CAD build for the part. Positions are in the model's coordinates, mm. Give positions to 0.01 mm unless a question says otherwise; leave off trailing zeros. Order: outer loops, then holes, each group sorted by start corner. A loop starts at its lowest first (then second) coordinate and runs counter-clockwise, first axis right, second up.
from build123d import *

# Parameters (mm, degrees)
BOSS_EXTRU_1_DEPTH = 2


with BuildPart() as part:
    # Esquisse1 → Boss.-Extru.1 (new body)
    with BuildSketch(Plane.XY):
        with BuildLine():
            Line((-875.748326024, -75.185778964), (-878.248326024, -75.185778964))
            Line((-878.248326024, -75.185778964), (-878.248326024, -67.185778964))
            Line((-878.248326024, -67.185778964), (-875.748326024, -67.185778964))
            Line((-875.748326024, -67.185778964), (-851.698326024, -67.185778964))
            ThreePointArc((-851.698326024, -67.185778964), (-849.970412013, -66.63818863), (-848.873290676, -65.195321078))
            Line((-848.873290676, -65.195321078), (-847.673290676, -61.837321078))
            ThreePointArc((-847.673290676, -61.837321078), (-847.542390805, -61.340074755), (-847.498326024, -60.827778964))
            Line((-847.498326024, -60.827778964), (-847.498326024, -56.827778964))
            ThreePointArc((-847.498326024, -56.827778964), (-847.538821892, -56.336520083), (-847.659216217, -55.858523838))
            Line((-847.659216217, -55.858523838), (-848.859216217, -52.343523838))
            ThreePointArc((-848.859216217, -52.343523838), (-849.95301307, -50.872721036), (-851.698326024, -50.312778964))
            Line((-851.698326024, -50.312778964), (-875.748326024, -50.312778964))
            Line((-875.748326024, -50.312778964), (-878.248326024, -50.312778964))
            Line((-878.248326024, -50.312778964), (-878.248326024, -40.935651694))
            Line((-878.248326024, -40.935651694), (-875.748326024, -40.935651694))
            Line((-875.748326024, -40.935651694), (-871.748326024, -40.935651694))
            Line((-871.748326024, -40.935651694), (-871.748326024, -31.558524425))
            Line((-871.748326024, -31.558524425), (-875.748326024, -31.558524425))
            Line((-875.748326024, -31.558524425), (-878.248326024, -31.558524425))
            Line((-878.248326024, -31.558524425), (-878.248326024, -22.181397155))
            Line((-878.248326024, -22.181397155), (-875.748326024, -22.181397155))
            Line((-875.748326024, -22.181397155), (-617.248326024, -22.181397155))
            Line((-617.248326024, -22.181397155), (-614.748326024, -22.181397155))
            Line((-614.748326024, -22.181397155), (-614.748326024, -31.558524425))
            Line((-614.748326024, -31.558524425), (-617.248326024, -31.558524425))
            Line((-617.248326024, -31.558524425), (-621.248326024, -31.558524425))
            Line((-621.248326024, -31.558524425), (-621.248326024, -40.935651694))
            Line((-621.248326024, -40.935651694), (-617.248326024, -40.935651694))
            Line((-617.248326024, -40.935651694), (-614.748326024, -40.935651694))
            Line((-614.748326024, -40.935651694), (-614.748326024, -50.312778964))
            Line((-614.748326024, -50.312778964), (-621.248326024, -50.312778964))
            Line((-621.248326024, -50.312778964), (-621.248326024, -67.185778964))
            Line((-621.248326024, -67.185778964), (-617.248326024, -67.185778964))
            Line((-617.248326024, -67.185778964), (-614.748326024, -67.185778964))
            Line((-614.748326024, -67.185778964), (-614.748326024, -75.185778964))
            Line((-614.748326024, -75.185778964), (-617.248326024, -75.185778964))
            Line((-617.248326024, -75.185778964), (-875.748326024, -75.185778964))
        make_face()
    extrude(amount=-BOSS_EXTRU_1_DEPTH)


solid = part.part
1. Wall check: line 1 (X direction, y = -35, z = -0.65); line 2 (X direction, y = -62, z = -1.2). Give the ranges that are in metal, low to high.
2. Saw through at B-B on z = -0.6. Give the cut face in (x, y), plus the area to 3 significant figures.
3. Pin check, flat tips, straight feed: P1, Ø0.6, axis at y = -36, z = -0.5, coming from the +X side; P2, Ø1, axis at y = -34, z = -1.5, coming from the -X side; P3, Ø0.6, axis at y = -59, z = -0.5, coming from the -X side. Stop position of each tip, or through.
4. Mould opens along Z. For faces 1 (the flat face through (-745, -48, -2)), 2 (the flat face through (-745, -48, 0)) say: released by +Z, released by -Z, zero draft, split by the parting line, or undercut.
5. Saw through at A-A on x = -860.5. Give the cut face in (y, z), plus the area to 3 significant figures.
Reported:
1. line 1: x = -871.75 to -621.25
1. line 2: x = -847.73 to -621.25
2. outline: (-878.25, -75.19) - (-614.75, -75.19) - (-614.75, -67.19) - (-621.25, -67.19) - (-621.25, -50.31) - (-614.75, -50.31) - (-614.75, -40.94) - (-621.25, -40.94) - (-621.25, -31.56) - (-614.75, -31.56) - (-614.75, -22.18) - (-878.25, -22.18) - (-878.25, -31.56) - (-871.75, -31.56) - (-871.75, -40.94) - (-878.25, -40.94) - (-878.25, -50.31) - (-851.7, -50.31) arc R3 cw to (-848.86, -52.34) - (-847.66, -55.86) arc R3 cw to (-847.5, -56.83) - (-847.5, -60.83) arc R3 cw to (-847.67, -61.84) - (-848.87, -65.2) arc R3 cw to (-851.7, -67.19) - (-878.25, -67.19) - close
2. area: 13,200 mm2
3. P1: stops at x = -621.25
3. P2: stops at x = -871.75
3. P3: stops at x = -847.5
4. face 1: released by -Z
4. face 2: released by +Z
5. outline: (-75.19, -2) - (-67.19, -2) - (-67.19, 0) - (-75.19, 0) - close; (-50.31, -2) - (-22.18, -2) - (-22.18, 0) - (-50.31, 0) - close
5. area: 72.3 mm2
